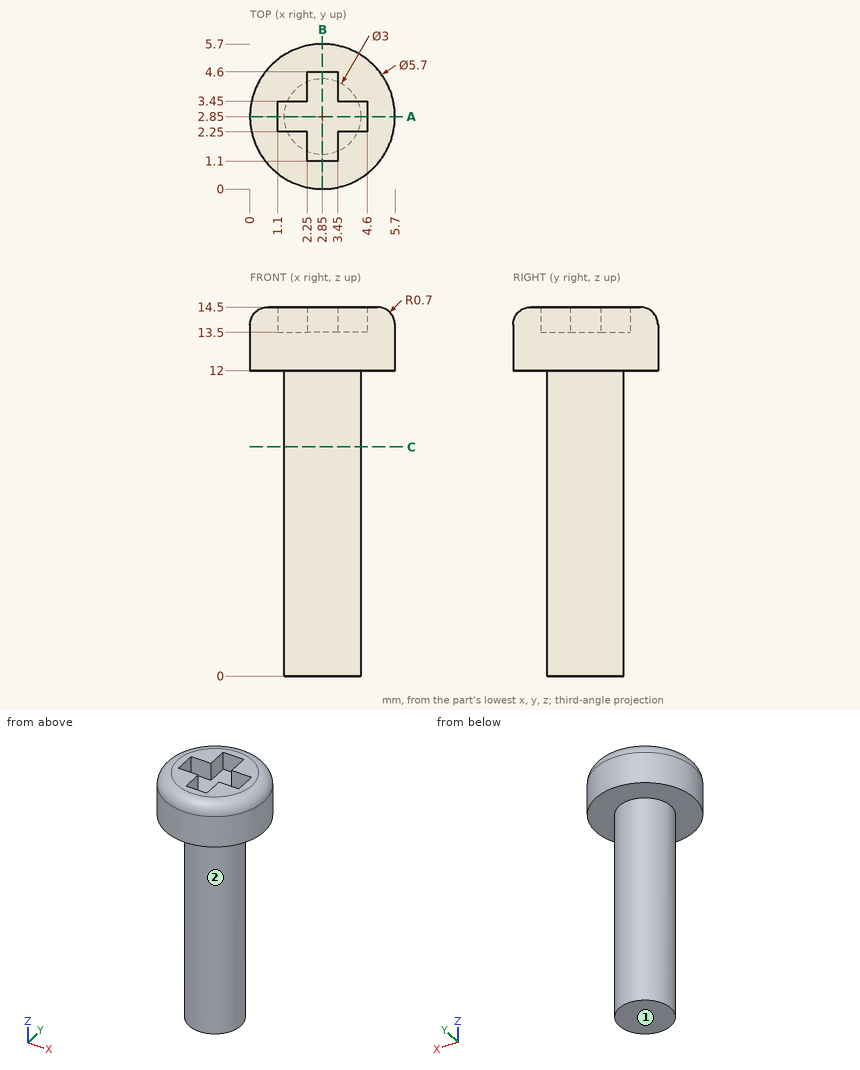
Study the drawing (mm; zero at the part's minimum x, y, z) and answer. A direction names the side the tool comes from. Give positions to 0.01 mm unless a question says otherwise; leave off trailing zeros. Write each loop counter-clockwise with the first axis right and the second up, starting at its lowest first coordinate (ties: lowest second). Pieces come first, ordered by that corner, then holes. Notation, with made-up numbers: (-32, 67) - (-8, 67) arc R17 cw to (-8, 82) - close; hole circle Ø6 at (38.5, -28). An arc over 180 degrees is marked (long way). Use a Markdown table: item, result.
1. Section C-C on z = 9 is taken. Write down the section's boundary in (x, y).
Values follow:
| item | result |
|---|---|
| outline | circle Ø3 at (2.85, 2.85) |
2. Each of these flat-tipped pins is pushed along its axis until it touches: P1, Ø1.7, axis at x = 2, y = 3, coming from the +Z side; P2, Ø0.8, axis at y = 1.5, z = 14, coming from the -X side; P3, Ø0.8, axis at y = 4, z = 14, coming from the +X side; P4, Ø3, axis at y = 1.5, z = 5, coming from the -X side. Where does it stop, or does it pass through?
Values follow:
| item | result |
|---|---|
| P1 | stops at z = 14.5 |
| P2 | stops at x = 0.17 |
| P3 | stops at x = 5.59 |
| P4 | stops at x = 1.35 |
3. Section A-A on y = 2.85 is taken. Write down the section's boundary in (x, z), plus the area to 3 significant figures.
Values follow:
| item | result |
|---|---|
| outline | (0, 12) - (1.35, 12) - (1.35, 0) - (4.35, 0) - (4.35, 12) - (5.7, 12) - (5.7, 13.8) arc R0.7 ccw to (5, 14.5) - (4.6, 14.5) - (4.6, 13.5) - (1.1, 13.5) - (1.1, 14.5) - (0.7, 14.5) arc R0.7 ccw to (0, 13.8) - close |
| area | 46.5 mm² |
4. A tool of negligible diameter and unlimited length cuts with its end or side. For the marked faces 1 and 2, from which of +Z, -Z, +X, -X, +Y, -Y can it reach the whole face along a straight path? Write none if from no direction.
Values follow:
| item | result |
|---|---|
| face 1 | -Z, +X, -X, +Y, -Y |
| face 2 | -Z |
5. Find the intervals of material crossed by probe 1 along Z at (x, y) = (1.55, 3.9); probe 2 along Z at (x, y) = (3.2, 2.9); probe 3 along X at (y, z) = (2.8, 6.25), in increasing order. Write a range as from..to.
Values follow:
| item | result |
|---|---|
| probe 1 | z = 12..14.5 |
| probe 2 | z = 0..13.5 |
| probe 3 | x = 1.35..4.35 |
